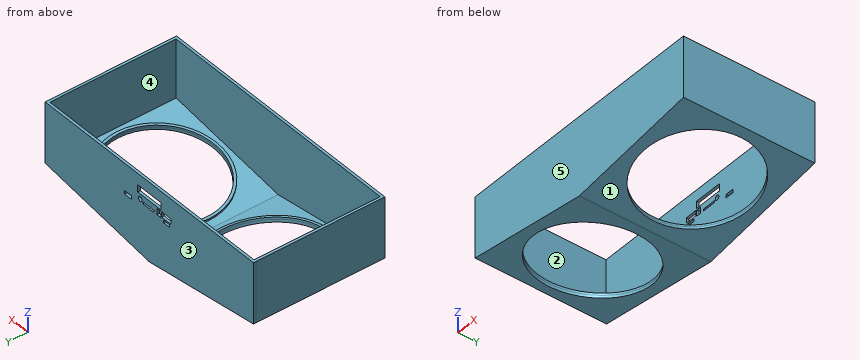
```python
from build123d import *

# Parameters (mm, degrees)
SALIENTE_EXTRUIR1_DEPTH = 145
CROQUIS3_R              = 66.25
CROQUIS3_R_2            = 63.25
SALIENTE_EXTRUIR2_DEPTH = 2.3
CROQUIS5_R              = 66.25
CROQUIS5_R_2            = 63.25
SALIENTE_EXTRUIR3_DEPTH = 2.3
CROQUIS6_R              = 63.25
CORTAR_EXTRUIR3_DEPTH   = 24.61469423
CROQUIS7_R              = 63.25
CORTAR_EXTRUIR4_DEPTH   = 24.61469423
SALIENTE_EXTRUIR4_DEPTH = 3
CROQUIS10_W             = 3
CROQUIS10_H             = 70
SALIENTE_EXTRUIR5_DEPTH = 148
SALIENTE_EXTRUIR6_DEPTH = 3
CROQUIS12_R             = 2.65
CROQUIS12_W             = 33.1
CROQUIS12_H             = 8.2
CROQUIS12_W_2           = 5.8
CROQUIS12_H_2           = 7.2
CROQUIS12_W_3           = 15.8
CROQUIS12_H_3           = 2.3
CROQUIS12_W_4           = 13.5
CROQUIS12_H_4           = 6
CROQUIS12_W_5           = 8.3
CROQUIS12_H_5           = 3
CROQUIS12_W_6           = 10
CROQUIS12_H_6           = 4
CORTAR_EXTRUIR5_DEPTH   = 10


with BuildPart() as part:
    # Croquis2 → Saliente-Extruir1 (new body)
    with BuildSketch(Plane(origin=(0, 0, 0), x_dir=(1, 0, 0), z_dir=(0, 1, 0))):
        Polygon((0, 90.302866191), (148.540210311, 69.426901047), (148.540210311, 72.456383764), (0.417519303, 93.273670397), (-0.417519303, 93.273670397), (-148.540210311, 72.456383764), (-148.540210311, 69.426901047), align=None)
    extrude(amount=SALIENTE_EXTRUIR1_DEPTH)

    # Croquis3 → Saliente-Extruir2 (add)
    with BuildSketch(Plane(origin=(12.44542163, 0, -88.553776247), x_dir=(0.990268069, 0, 0.139173101), z_dir=(-0.139173101, 0, 0.990268069))):
        with Locations((62.432270087, 72.5)):
            Circle(CROQUIS3_R)
        with Locations((62.432270087, 72.5)):
            Circle(CROQUIS3_R_2, mode=Mode.SUBTRACT)
    extrude(amount=SALIENTE_EXTRUIR2_DEPTH)

    # Croquis5 → Saliente-Extruir3 (add)
    with BuildSketch(Plane(origin=(-12.44542163, 0, -88.553776247), x_dir=(0.990268069, 0, -0.139173101), z_dir=(0.139173101, 0, 0.990268069))):
        with Locations((-62.432270087, 72.5)):
            Circle(CROQUIS5_R)
        with Locations((-62.432270087, 72.5)):
            Circle(CROQUIS5_R_2, mode=Mode.SUBTRACT)
    extrude(amount=SALIENTE_EXTRUIR3_DEPTH)

    # Croquis6 → Cortar-Extruir3 (cut, through all)
    with BuildSketch(Plane(origin=(-12.44542163, 0, -88.553776247), x_dir=(0.990268069, 0, -0.139173101), z_dir=(0.139173101, 0, 0.990268069))):
        with Locations((-62.432270087, 72.5)):
            Circle(CROQUIS6_R)
    extrude(amount=-CORTAR_EXTRUIR3_DEPTH, mode=Mode.SUBTRACT)

    # Croquis7 → Cortar-Extruir4 (cut, through all)
    with BuildSketch(Plane(origin=(12.44542163, 0, -88.553776247), x_dir=(0.990268069, 0, 0.139173101), z_dir=(-0.139173101, 0, 0.990268069))):
        with Locations((62.432270087, 72.5)):
            Circle(CROQUIS7_R)
    extrude(amount=-CORTAR_EXTRUIR4_DEPTH, mode=Mode.SUBTRACT)

    # Croquis9 → Saliente-Extruir4 (add)
    with BuildSketch(Plane.XZ):
        Polygon((-148.540210311, -72.456383764), (-0.417519303, -93.273670397), (0.417519303, -93.273670397), (148.540210311, -72.456383764), (148.540210311, -2.456383764), (-148.540210311, -2.456383764), align=None)
    extrude(amount=SALIENTE_EXTRUIR4_DEPTH)

    # Croquis10 → Saliente-Extruir5 (add)
    with BuildSketch(Plane.XZ.offset(3)):
        with Locations((-147.040210311, -37.456383764)):
            Rectangle(CROQUIS10_W, CROQUIS10_H)
        with Locations((147.040210311, -37.456383764)):
            Rectangle(CROQUIS10_W, CROQUIS10_H)
    extrude(amount=-SALIENTE_EXTRUIR5_DEPTH)

    # Croquis11 → Saliente-Extruir6 (add)
    with BuildSketch(Plane(origin=(0, 145, 0), x_dir=(1, 0, 0), z_dir=(0, 1, 0))):
        Polygon((148.540210311, 72.456383764), (0.417519303, 93.273670397), (-0.417519303, 93.273670397), (-148.540210311, 72.456383764), (-148.540210311, 2.456383764), (148.540210311, 2.456383764), align=None)
    extrude(amount=SALIENTE_EXTRUIR6_DEPTH)

    # Croquis12 → Cortar-Extruir5 (cut)
    with BuildSketch(Plane.XZ.offset(-145)):
        with Locations((12.9, -29.517649177)):
            Circle(CROQUIS12_R)
        with Locations((0, -19.556383764)):
            Rectangle(CROQUIS12_W, CROQUIS12_H)
        with Locations((-13.65, -28.956383764)):
            Rectangle(CROQUIS12_W_2, CROQUIS12_H_2)
        with Locations((1.15, -31.506383764)):
            Rectangle(CROQUIS12_W_3, CROQUIS12_H_3)
        with Locations((-24.3, -28.356383764)):
            Rectangle(CROQUIS12_W_4, CROQUIS12_H_4)
        with Locations((-24.3, -34.656383764)):
            Rectangle(CROQUIS12_W_5, CROQUIS12_H_5)
        with Locations((30.45, -35.656383764)):
            Rectangle(CROQUIS12_W_6, CROQUIS12_H_6)
    extrude(amount=-CORTAR_EXTRUIR5_DEPTH, mode=Mode.SUBTRACT)


solid = part.part
```
Design review of the part built by this model. Coordinates are the model's own, in mm. Face numbers are marked on the shaded views. A direction names the side the tool comes from. Give positions to 0.01 mm unless a question says otherwise; leave off trailing zeros. Write each loop counter-clockwise with the first axis right and the second up, starting at its lowest first coordinate (ties: lowest second). Pieces come first, ordered by that corner, then holes. Notation, with made-up numbers: (3, 9) - (52, 9) arc R18 ccw to (52, 18) - close; hole circle Ø5 at (21, -37.75). An arc over 180 degrees is marked (long way). Return JSON: item names as keys, results as strings. Group by question number.
(1) We need section A-A, the plane y = 35. Give the boundary of the cut face in (x, z), then the cut area to 3 significant figures.
(2) We need section C-C, the plane y = 90.5. Give the boundary of the cut face in (x, z).
(3) Mouldability with a two-part tool opening along Y and no side actions: class the marked faces 3, 4 and 5 as +Y half, -Y half, draft (parallel to the pull), parting line (faces both ways), or undercut.
(4) Insertion check: pin 1 (1.5 mm diameter, centred on x = -5.5, y = 147, fed in from -Z); pin 2 (0.9 mm diameter, centred on x = 32, y = 147, fed in from -Z); pin 3 (3.5 mm diameter, centred on x = -23, y = 147, fed in from -Z). Each pin has a flat end and moves straight along its axis. Give the tip position at first contact, or say it passes through.
(5) We need section B-B, the plane z = -48. Give the boundary of the cut face in (x, y).
(6) To check wall thickness, follow probe 1 along X at (y, z) = (141, -60.5); probe 2 along Y at (x, z) = (-100, -8); probe 3 along Z at (x, y) = (12, 146). State the ranges of each line that lie inside material, in increasing order.
(7) Machinability: for the marked faces 1 and 2, which of the approach directions +Z, -Z, +X, -X, +Y, -Y give a long, thin tool a straight path to every point of the face, cutting with its end or side? Answer none if there is none.
Reported:
{
 "1": {"outline": "(-148.54, -72.46) - (-125.13, -75.75) - (-124.39, -70.5) - (-128.03, -69.99) - (-128.35, -72.26) - (-145.54, -69.85) - (-145.54, -2.46) - (-148.54, -2.46) - close; (-24.25, -89.92) - (-0.42, -93.27) - (0.42, -93.27) - (24.25, -89.92) - (23.51, -84.68) - (19.87, -85.19) - (20.19, -87.47) - (0, -90.3) - (-20.19, -87.47) - (-19.87, -85.19) - (-23.51, -84.68) - close; (124.39, -70.5) - (125.13, -75.75) - (148.54, -72.46) - (148.54, -2.46) - (145.54, -2.46) - (145.54, -69.85) - (128.35, -72.26) - (128.03, -69.99) - close", "area": "726 mm2"},
 "2": {"outline": "(-148.54, -72.46) - (-134.73, -74.4) - (-133.99, -69.15) - (-137.09, -68.71) - (-137.41, -70.99) - (-145.54, -69.85) - (-145.54, -2.46) - (-148.54, -2.46) - close; (-14.64, -91.27) - (-0.42, -93.27) - (0.42, -93.27) - (14.64, -91.27) - (13.91, -86.03) - (10.81, -86.46) - (11.13, -88.74) - (0, -90.3) - (-11.13, -88.74) - (-10.81, -86.46) - (-13.91, -86.03) - close; (133.99, -69.15) - (134.73, -74.4) - (148.54, -72.46) - (148.54, -2.46) - (145.54, -2.46) - (145.54, -69.85) - (137.41, -70.99) - (137.09, -68.71) - close"},
 "3": {"face 3": "+Y half", "face 4": "undercut", "face 5": "-Y half"},
 "4": {"pin 1": "stops at z = -92.66", "pin 2": "stops at z = -88.9", "pin 3": "stops at z = -90.35"},
 "5": {"outline": "(-148.54, -3) - (148.54, -3) - (148.54, 148) - (-148.54, 148) - close; hole (-145.54, 0) - (145.54, 0) - (145.54, 145) - (-145.54, 145) - close"},
 "6": {"probe 1": "x = -148.54 to -145.54, 145.54 to 148.54", "probe 2": "y = -3 to 0, 145 to 148", "probe 3": "z = -91.65 to -32.01, -27.03 to -23.66, -15.46 to -2.46"},
 "7": {"face 1": "-Z, +X, +Y, -Y", "face 2": "+Z"}
}
